The listing builds one solid part. Answer for the finished solid, in the listing's coordinates (mm). Give positions to 0.01 mm unless a question says otherwise; leave off trailing zeros. Loops run counter-clockwise (first coordinate to the right, second up) from the corner with the lowest first, then second, coordinate; pieces in that order, holes last. Notation, with made-up numbers: (70.5, -29.75) - (110.5, -29.75) arc R19 ccw to (110.5, -15.75) - close; hole circle Ø3 at (69, -35). An arc over 180 degrees is marked (long way). Write item = value, one per line. Start each with the question number.
1) The part is cut by section A-A on x = -5. Write down the section's boundary in (y, z), plus the area to 3 significant figures.
2) Consider probe 1 along Y at (x, z) = (-10, 1.2); probe 2 along Y at (x, z) = (-11, 0.95); probe 3 along X at (y, z) = (-28, 0.9). Determine where each line is inside the solid, lowest interval first.
3) The mould has two halves that part along X. Classify faces 1 (the flat face through (-8, -15, 2)), 2 (the flat face through (-30, 0, 1)), 3 (the cylindrical face through (-16.5, 0.07, 0.99)): +X half, -X half, draft (parallel to the pull), parting line (faces both ways), or undercut.
4) The part is cut by section D-D on y = 0. Write down the section's boundary in (x, z).
5) The part is cut by section C-C on z = 0.75. Write down the section's boundary in (x, y), plus the area to 3 significant figures.
6) The part is cut by section B-B on y = -30. Write down the section's boundary in (x, z).
from build123d import *

# Parameters (mm, degrees)
SKETCH_1_R      = 1.5
EXTRUDE_1_DEPTH = 2
FILLET_1_R      = 1


with BuildPart() as part:
    # 草图1 → 凸台-拉伸1 (new body)
    with BuildSketch(Plane.XY):
        Polygon((-30, -5), (-30, 5), (5, 5), (5, -35), (-15, -35), align=None)
        with Locations((-15, 0)):
            Circle(SKETCH_1_R, mode=Mode.SUBTRACT)
        with Locations((-5, 0)):
            Circle(SKETCH_1_R, mode=Mode.SUBTRACT)
        with Locations((-10, -15)):
            Circle(SKETCH_1_R, mode=Mode.SUBTRACT)
        with Locations((-10, -30)):
            Circle(SKETCH_1_R, mode=Mode.SUBTRACT)
        with Locations((0, -30)):
            Circle(SKETCH_1_R, mode=Mode.SUBTRACT)
        with Locations((0, -15)):
            Circle(SKETCH_1_R, mode=Mode.SUBTRACT)
    extrude(amount=EXTRUDE_1_DEPTH)

    # 圆角1
    fillet_1_edges = [part.edges().sort_by_distance(p)[0] for p in [
        (-30, -5, 1),
        (-30, 5, 1),
        (5, 5, 1),
        (5, -35, 1),
        (-15, -35, 1),
    ]]
    fillet(fillet_1_edges, radius=FILLET_1_R)


solid = part.part
Answer below:
q1.outline = (-35, 0) - (-1.5, 0) - (-1.5, 2) - (-35, 2) - close; (1.5, 0) - (5, 0) - (5, 2) - (1.5, 2) - close
q1.area = 74.0 mm2
q2.probe_1 = -35 to -31.5, -28.5 to -16.5, -13.5 to 5
q2.probe_2 = -35 to -31.12, -28.88 to -16.12, -13.88 to 5
q2.probe_3 = -18.5 to 5
q3.face_1 = draft
q3.face_2 = -X half
q3.face_3 = undercut
q4.outline = (-30, 0) - (-16.5, 0) - (-16.5, 2) - (-30, 2) - close; (-13.5, 0) - (-6.5, 0) - (-6.5, 2) - (-13.5, 2) - close; (-3.5, 0) - (5, 0) - (5, 2) - (-3.5, 2) - close
q5.outline = (-30, -4.76) arc R1 ccw to (-29.89, -5.21) - (-15.28, -34.45) arc R1 ccw to (-14.38, -35) - (4, -35) arc R1 ccw to (5, -34) - (5, 4) arc R1 ccw to (4, 5) - (-29, 5) arc R1 ccw to (-30, 4) - close; hole circle Ø3 at (-15, 0); hole circle Ø3 at (-10, -30); hole circle Ø3 at (-10, -15); hole circle Ø3 at (-5, 0); hole circle Ø3 at (0, -30); hole circle Ø3 at (0, -15)
q5.area = 1,130 mm2
q6.outline = (-17.5, 0) - (-11.5, 0) - (-11.5, 2) - (-17.5, 2) - close; (-8.5, 0) - (-1.5, 0) - (-1.5, 2) - (-8.5, 2) - close; (1.5, 0) - (5, 0) - (5, 2) - (1.5, 2) - close
